CAD build for the part. Positions are in the model's coordinates, mm. Face numbers are marked on the shaded views. Give positions to 0.01 mm unless a question says otherwise; leave off trailing zeros. Loops run counter-clockwise (first coordinate to the right, second up) from the corner with the lowest first, then second, coordinate; pieces in that order, holes last. Notation, with made-up numbers: M -2.5,63.25 L 45.5,63.25 A26 ccw 45.5,96.25 Z; hole C 34.5,-24 d8. An arc over 180 degrees is marked long. One line per question, with ' | ' between items.
```python
from build123d import *

# Parameters (mm, degrees)
SKETCH1_W                                    = 110
SKETCH1_H                                    = 30
EXTRUDE1_DEPTH                               = 2
CUT_EXTRUDE1_DEPTH                           = 3
CHAMFER1_SIZE                                = 9
CHAMFER1_SIZE2                               = 1.5
CSK_FOR_M3_COUNTERSUNK_RAISED_HEAD_S_2_COUNT = 2
CSK_FOR_M3_COUNTERSUNK_RAISED_HEAD_S_2_PITCH = 95
CSK_FOR_M3_COUNTERSUNK_RAISED_HEAD_S_3_COUNT = 2
CSK_FOR_M3_COUNTERSUNK_RAISED_HEAD_S_3_PITCH = 97.082439195
CSK_FOR_M3_COUNTERSUNK_RAISED_HEAD_S_4_COUNT = 2
CSK_FOR_M3_COUNTERSUNK_RAISED_HEAD_S_4_PITCH = 20
M3_TAPPED_HOLE1_D                            = 3
SKETCH13_R                                   = 30.96323942
CUT_EXTRUDE2_DEPTH                           = 3


with BuildPart() as part:
    # Sketch1 → Extrude1 (new body)
    with BuildSketch(Plane(origin=(0, 0, 0), x_dir=(1, 0, 0), z_dir=(0, 1, 0))):
        Rectangle(SKETCH1_W, SKETCH1_H)
    extrude(amount=EXTRUDE1_DEPTH)

    # Sketch2 → Cut-Extrude1 (cut, through all)
    with BuildSketch(Plane(origin=(0, 2, 0), x_dir=(-1, 0, 0), z_dir=(0, 1, 0))):
        with BuildLine():
            Line((5, 0), (5, -15))
            Line((5, -15), (-5, -15))
            Line((-5, -15), (-5, 0))
            ThreePointArc((-5, 0), (0, 5), (5, 0))
        make_face()
    extrude(amount=-CUT_EXTRUDE1_DEPTH, mode=Mode.SUBTRACT)

    # Chamfer1
    chamfer1_edges = [part.edges().sort_by_distance(p)[0] for p in [
        (0, 2, 5),
        (5, 2, -7.5),
        (-5, 2, -7.5),
    ]]
    chamfer1_side = [part.faces().sort_by_distance(p)[0] for p in [
        (-53.859824575, 2, 0),
    ]]
    chamfer(chamfer1_edges, length=CHAMFER1_SIZE, length2=CHAMFER1_SIZE2, reference=chamfer1_side[0])

    # Sketch8 → CSK for M3 Countersunk Raised Head Screw1 (revolve, cut)
    with BuildSketch(Plane(origin=(47.5, 0, -10), x_dir=(0, 0, -1), z_dir=(1, 0, 0))):
        Polygon((0, 0), (0, 2), (1.7, 2), (1.7, 1.45), (3.15, 0), align=None)
    csk_for_m3_countersunk_raised_head_screw = revolve(axis=Axis((47.5, -6.35, -10), (0, 1, 0)), mode=Mode.SUBTRACT)

    # CSK for M3 Countersunk Raised Head S 2: CSK for M3 Countersunk Raised Head Screw1 ×2
    with Locations(*[(-i * CSK_FOR_M3_COUNTERSUNK_RAISED_HEAD_S_2_PITCH, 0, 0) for i in range(1, CSK_FOR_M3_COUNTERSUNK_RAISED_HEAD_S_2_COUNT)]):
        add(csk_for_m3_countersunk_raised_head_screw, mode=Mode.SUBTRACT)

    # CSK for M3 Countersunk Raised Head S 3: CSK for M3 Countersunk Raised Head Screw1 ×2
    with Locations(*[Vector(-0.978549785, 0, 0.206010481) * (i * CSK_FOR_M3_COUNTERSUNK_RAISED_HEAD_S_3_PITCH) for i in range(1, CSK_FOR_M3_COUNTERSUNK_RAISED_HEAD_S_3_COUNT)]):
        add(csk_for_m3_countersunk_raised_head_screw, mode=Mode.SUBTRACT)

    # CSK for M3 Countersunk Raised Head S 4: CSK for M3 Countersunk Raised Head Screw1 ×2
    with Locations(*[(0, 0, i * CSK_FOR_M3_COUNTERSUNK_RAISED_HEAD_S_4_PITCH) for i in range(1, CSK_FOR_M3_COUNTERSUNK_RAISED_HEAD_S_4_COUNT)]):
        add(csk_for_m3_countersunk_raised_head_screw, mode=Mode.SUBTRACT)

    # M3 Tapped Hole1 (through all)
    with Locations(Plane(origin=(0, 2, 0), x_dir=(-1, 0, 0), z_dir=(0, 1, 0))):
        with Locations((-30, 0), (30, 0)):
            Hole(M3_TAPPED_HOLE1_D / 2)

    # Sketch13 → Cut-Extrude2 (cut, through all)
    with BuildSketch(Plane.XZ):
        with Locations((0, -32.270962356)):
            Circle(SKETCH13_R)
    extrude(amount=-CUT_EXTRUDE2_DEPTH, mode=Mode.SUBTRACT)


solid = part.part
```
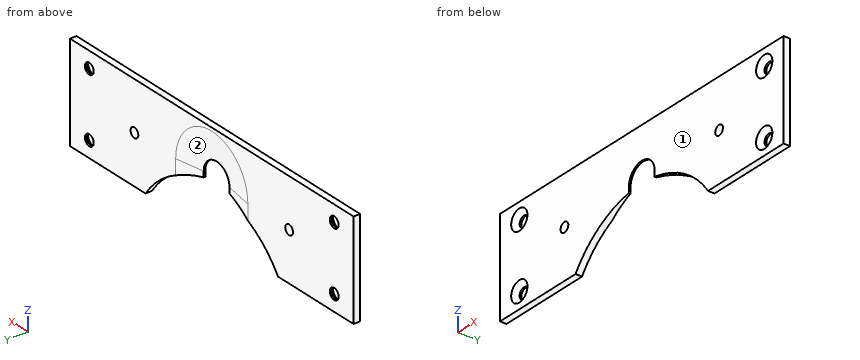
Item 1: Saw through at D-D on y = 1. Give the cut face in (x, z), and give its area (3 significant figures).
Conclusion:
outline: M -55,-15 L -25.7,-15 A30.96 cw -8,-2.36 L -8,0 A8 cw 8,0 L 8,-2.36 A30.96 cw 25.7,-15 L 55,-15 L 55,15 L -55,15 Z; hole C -47.5,-10 d4.3; hole C -47.5,10 d4.3; hole C -30,0 d3; hole C 30,0 d3; hole C 47.5,-10 d4.3; hole C 47.5,10 d4.3 | area: 2,610 mm²
Item 2: Saw through at C-C on x = 30. Give the cut face in (y, z).
Conclusion:
outline: M 0,-15 L 2,-15 L 2,-1.5 L 0,-1.5 Z; M 0,1.5 L 2,1.5 L 2,15 L 0,15 Z
Item 3: Saw through at B-B on z = -10. Give the cut face in (x, y).
Conclusion:
outline: M -55,0 L -50.65,0 L -49.2,1.45 L -49.2,2 L -55,2 Z; M -45.8,1.45 L -44.35,0 L -21.51,0 L -21.51,2 L -45.8,2 Z; M 21.51,0 L 44.35,0 L 45.8,1.45 L 45.8,2 L 21.51,2 Z; M 49.2,1.45 L 50.65,0 L 55,0 L 55,2 L 49.2,2 Z
Item 4: Mould opens along X. For the marked faces 1 and 2 say: pulls with the +X half, pulls with the -X half, needs draft (parallel to the pull), parting line crosses it, or undercut.
Conclusion:
face 1: needs draft | face 2: undercut
Item 5: Saw through at A-A on x = 47.5. Give the cut face in (y, z), and give its area (3 significant figures).
Conclusion:
outline: M 0,-15 L 2,-15 L 2,-11.7 L 1.45,-11.7 L 0,-13.15 Z; M 0,-6.85 L 1.45,-8.3 L 2,-8.3 L 2,8.3 L 1.45,8.3 L 0,6.85 Z; M 0,13.15 L 1.45,11.7 L 2,11.7 L 2,15 L 0,15 Z | area: 42.2 mm²
Item 6: Drill centre lines: line 1 along Z through (x, y) = (47.5, 1.75); line 2 along X through (y, z) = (1.9, -10); line 3 along Z through (x, y) = (-30, 1.4). Where is each one in solid material? Low to high. Write a range as [from, to].
Conclusion:
line 1: [-15, -11.7], [-8.3, 8.3], [11.7, 15] | line 2: [-55, -49.2], [-45.8, -21.51], [21.51, 45.8], [49.2, 55] | line 3: [-15, -1.5], [1.5, 15]
Item 7: Drop flat-ended pins along their axis: P1, Ø4.5, axis at x = -47.5, z = -10, coming from the -Y side; P2, Ø4, axis at x = -47.5, z = 10, coming from the +Y side; P3, Ø12, axis at x = -7, z = -2.5, coming from the +Y side. Give the stop position or say it passes through.
Conclusion:
P1: y = 0.9 | P2: y = 2 | P3: y = 1.83
